Autodesk Inventor part; units mm, degrees
ref_plane "YZ Plane" through (0, 0, 0) normal (1, 0, 0) x (0, 1, 0)
ref_plane "XZ Plane" through (0, 0, 0) normal (0, 1, 0) x (-1, 0, 0)
ref_plane "XY Plane" through (0, 0, 0) normal (0, 0, 1) x (1, 0, 0)
sketch "Sketch1" plane through (0, 0, 0) normal (0, 0, 1) x (1, 0, 0)
  line L0 (2.54, 0) -> (15.24, 0)
  line L1 (17.78, 2.54) -> (17.78, 22.86)
  line L2 (15.24, 25.4) -> (2.54, 25.4)
  line L3 (0, 22.86) -> (0, 2.54)
  arc A0 (17.78, 22.86) -> (15.24, 25.4) centre (15.24, 22.86) ccw
  arc A1 (15.24, 0) -> (17.78, 2.54) centre (15.24, 2.54) ccw
  arc A2 (0, 2.54) -> (2.54, 0) centre (2.54, 2.54) ccw
  arc A3 (2.54, 25.4) -> (0, 22.86) centre (2.54, 22.86) ccw
  point P0 (0, 0)
  point P1 (17.78, 25.4)
  point P2 (17.78, 0)
  point P3 (0, 25.4)
  dimension "d0" = 17.78
  dimension "d1" = 25.4
  dimension "d2" = 2.54
extrude "Extrusion1" add sketch "Sketch1" along normal blind 1.5367
sketch "Sketch2" plane through (0, 0, 1.5367) normal (0, 0, 1) x (1, 0, 0)
  arc A0 (17.78, 22.86) -> (15.24, 25.4) centre (15.24, 22.86) ccw
  arc A1 (15.24, 0) -> (17.78, 2.54) centre (15.24, 2.54) ccw
  line L0 (17.78, 2.54) -> (17.78, 22.86)
  line L1 (15.24, 25.4) -> (2.54, 25.4)
  line L2 (2.54, 0) -> (15.24, 0)
  point P0 (0, 0)
  point P1 (15.1511, 22.7711)
  point P2 (15.1511, 2.6289)
  dimension "d36" = 2.6289
  dimension "d37" = 2.6289
  dimension "d38" = 2.6289
  dimension "d39" = 2.6289
hole "Hole1" at (15.1511, 22.7711, 1.5367) at (15.1511, 2.6289, 1.5367) direction (0, 0, -1) diameter 2.4638 end through all both
sketch "Sketch3" plane through (0, 0, 1.5367) normal (0, 0, 1) x (1, 0, 0)
  arc A0 (17.78, 22.86) -> (15.24, 25.4) centre (15.24, 22.86) ccw construction
  line L0 (15.24, 25.4) -> (15.24, 0) construction
  arc A1 (15.24, 0) -> (17.78, 2.54) centre (15.24, 2.54) ccw construction
  line L1 (2.54, 0) -> (15.24, 0) construction
  line L2 (15.24, 25.4) -> (2.54, 25.4) construction
  line L3 (2.54, 0) -> (2.54, 25.4) construction
  line L4 (0, 22.86) -> (0, 2.54) construction
  line L5 (0, 12.7) -> (17.78, 12.7) construction
  line L6 (17.78, 2.54) -> (17.78, 22.86) construction
  line L7 (8.89, 25.4) -> (8.89, 0) construction
  point P0 (0, 0)
  point P1 (15.24, 13.97)
  point P2 (2.54, 13.97)
  point P3 (15.24, 16.51)
  point P4 (15.24, 19.05)
  point P5 (15.24, 11.43)
  point P6 (15.24, 13.97)
  point P7 (15.24, 16.51)
  point P8 (15.24, 8.89)
  point P9 (15.24, 11.43)
  point P10 (15.24, 13.97)
  point P11 (15.24, 6.35)
  point P12 (15.24, 8.89)
  point P13 (15.24, 11.43)
  point P14 (2.54, 16.51)
  point P15 (2.54, 19.05)
  point P16 (2.54, 21.59)
  point P17 (2.54, 11.43)
  point P18 (2.54, 13.97)
  point P19 (2.54, 16.51)
  point P20 (2.54, 19.05)
  point P21 (2.54, 8.89)
  point P22 (2.54, 11.43)
  point P23 (2.54, 13.97)
  point P24 (2.54, 16.51)
  point P25 (2.54, 6.35)
  point P26 (2.54, 8.89)
  point P27 (2.54, 11.43)
  point P28 (2.54, 13.97)
  point P29 (2.54, 3.81)
  point P30 (2.54, 6.35)
  point P31 (2.54, 8.89)
  point P32 (2.54, 11.43)
  dimension "d12" = 1.27
  dimension "d15" = 2.54
  dimension "d18" = 2.54
  dimension "d23" = 2.54
  dimension "d26" = 2.54
hole "Hole2" at (15.24, 13.97, 1.5367) at (2.54, 13.97, 1.5367) at (15.24, 16.51, 1.5367) at (15.24, 19.05, 1.5367) at (15.24, 11.43, 1.5367) at (15.24, 8.89, 1.5367) at (15.24, 6.35, 1.5367) at (2.54, 16.51, 1.5367) at (2.54, 19.05, 1.5367) at (2.54, 21.59, 1.5367) at (2.54, 11.43, 1.5367) at (2.54, 8.89, 1.5367) at (2.54, 6.35, 1.5367) at (2.54, 3.81, 1.5367) direction (0, 0, -1) diameter 1.016 end through all both
equation "\"d3\" = pcbThickness"
equation "\"d5\" = mountingHoleDiameter"
equation "\"d29\" = pinHoleDiameter"
equation "\"pcbThickness\" = 1.5367"
equation "\"mountingHoleDiameter\" = 2.4638"
equation "\"pinHoleDiameter\" = 1.016"
equation "\"pinHoleSeparationDistance\" = 2.54"
properties part number "Driver_Motor"
The model under review builds one solid part; all positions refer to its coordinate system, in mm. Round coordinates to 2 decimals unless told otherwise and drop trailing zeros. Loops run counter-clockwise (first coordinate to the right, second up) from the corner with the lowest first, then second, coordinate; pieces in that order, holes last.
1) Clearance check with flat-ended pins moving along their axes: P1, Ø0.9, axis at x = 2.54, y = 19.05, coming from the -Z side; P2, Ø4, axis at x = 15.15, y = 22.77, coming from the -Z side. State where each tip first meets the part, or that it passes through.
Values follow:
P1: passes through
P2: stops at z = 0
2) Wall thickness on line 1 along X through (y, z) = (19.05, 0.4); line 2 along X through (y, z) = (16.75, 1.15); line 3 along Y through (x, z) = (16, 0.1): over which ranges is each line inside the solid? List them lowest first.
Values follow:
line 1: x = 0 to 2.03, 3.05 to 14.73, 15.75 to 17.78
line 2: x = 0 to 2.09, 2.99 to 14.79, 15.69 to 17.78
line 3: y = 0.12 to 1.74, 3.52 to 21.88, 23.66 to 25.28
3) The part is to be moulded in two halves that separate along Y. For faces 1 (the face through (0.764, 0.724, 0.758)), 2 (the face through (15.9, 23.75, 0.76)), 3 (the face through (14.897, 14.344, 0.758)), 4 (the face through (0, 13, 1)), say which applies: pulls with the +Y half, pulls with the -Y half, needs draft (parallel to the pull), parting line crosses it, or undercut.
Values follow:
face 1: pulls with the -Y half
face 2: undercut
face 3: undercut
face 4: needs draft
4) Consider section B-B on y = 3. State the section outline as (x, z) points.
Values follow:
outline: (0, 0) - (13.98, 0) - (13.98, 1.54) - (0, 1.54) - close; (16.33, 0) - (17.78, 0) - (17.78, 1.54) - (16.33, 1.54) - close
5) Consider section A-A on y = 19.05. State the section outline as (x, z) points.
Values follow:
outline: (0, 0) - (2.03, 0) - (2.03, 1.54) - (0, 1.54) - close; (3.05, 0) - (14.73, 0) - (14.73, 1.54) - (3.05, 1.54) - close; (15.75, 0) - (17.78, 0) - (17.78, 1.54) - (15.75, 1.54) - close
6) Consider section C-C on z = 0.3. Give the number of separate pieces and of enclosed holes in the cut face, then the cut area to 3 significant figures.
Values follow:
separate pieces: 1
enclosed holes: 16
area: 425 mm2
